from build123d import *

# Parameters (mm, degrees)
SKETCH1_W           = 36.310674736
SKETCH1_H           = 16.43794059
BOSS_EXTRUDE1_DEPTH = 2.54
FILLET1_R           = 2.54
FILLET2_R           = 2.54


# Some blends are built 0.0001 mm under size
with BuildPart() as part:
    # Sketch1 → Boss-Extrude1 (new body)
    with BuildSketch(Plane(origin=(0, 0, 0), x_dir=(1, 0, 0), z_dir=(0, 1, 0))):
        Rectangle(SKETCH1_W, SKETCH1_H)
    extrude(amount=BOSS_EXTRUDE1_DEPTH)

    # Fillet1
    fillet1_edges = [part.edges().sort_by_distance(p)[0] for p in [
        (18.155337368, 1.27, 8.218970295),
        (-18.155337368, 1.27, 8.218970295),
        (0, 2.54, 8.218970295),
    ]]
    fillet(fillet1_edges, radius=FILLET1_R - 0.0001)  # a hair under: the kernel refuses the full size

    # Fillet2
    # the kernel refuses this fillet: 2.54 mm, written as the material it takes off along each edge
    with BuildSketch(Plane(origin=(-15.615337368, 0, 8.218970295), x_dir=(0, 1, 0), z_dir=(1, 0, 0))) as fillet2_piece_1:
        with BuildLine():
            CenterArc((0.0001, -2.5399), 2.5399, 0, 90)
            Line((2.54, -2.5399), (2.54, 0))
            Line((2.54, 0), (0.0001, 0))
        make_face()
    revolve(axis=Axis((-15.615337368, 0, 8.218970295), (0, 0, 1)), revolution_arc=90, mode=Mode.SUBTRACT)
    with BuildSketch(Plane(origin=(15.615337368, 0, 8.218970295), x_dir=(1, 0, 0), z_dir=(0, -1, 0))) as fillet2_piece_2:
        with BuildLine():
            CenterArc((0.0001, -2.5399), 2.5399, 0, 90)
            Line((2.54, -2.5399), (2.54, 0))
            Line((2.54, 0), (0.0001, 0))
        make_face()
    revolve(axis=Axis((15.615337368, 0, 8.218970295), (0, 0, 1)), revolution_arc=90, mode=Mode.SUBTRACT)
    with BuildSketch(Plane(origin=(-18.155337368, 2.54, 8.218970295), x_dir=(0, -1, 0), z_dir=(0, 0, -1)), Plane(origin=(18.155337368, 2.54, -14.568970295), x_dir=(0, -1, 0), z_dir=(0, 0, 1))) as fillet2_piece_3:
        with BuildLine():
            CenterArc((FILLET2_R, -FILLET2_R), FILLET2_R, 90, 90)
            Line((0, -FILLET2_R), (0, 0))
            Line((0, 0), (FILLET2_R, 0))
        make_face()
    extrude(amount=22.78794059, mode=Mode.SUBTRACT)


solid = part.part
Could you check a few things on this model? Use its own coordinates, in mm. Give positions to 0.01 mm unless a question says otherwise; leave off trailing zeros. Write each loop counter-clockwise with the first axis right and the second up, starting at its lowest first coordinate (ties: lowest second). Pieces come first, ordered by that corner, then holes. Notation, with made-up numbers: (-1.75, 88.5) -> (14.25, 88.5) arc R18 cw to (14.25, 109.5) -> close; hole circle Ø7 at (18.5, 71). An arc over 180 degrees is marked (long way). Answer as CSV lines item,"result". Start each with the question number.
(1) Please list where these lines run through material, in increasing order: line 1 (Y direction, x = -15.5, z = 5.75); line 2 (Z direction, x = -9, y = 2.3); line 3 (Z direction, x = 1, y = 2.1).
(2) If we section it at B-B, the plane z = -6: Write out the boundary of the cut face in (x, y).
(3) I'm going to push flat-ended pins straight in: pin 1 Ø1.5 at (y, z) = (2.5, 2.5) entering from -X; pin 2 Ø1 at (x, y) = (3, 1.5) entering from +Z. Where does each tip first touch, or does it pass through?
Answer list:
1,line 1,"0 to 2.54"
1,line 2,"-8.22 to 6.76"
1,line 3,"-8.22 to 7.11"
2,outline,"(-18.16, 0) -> (18.16, 0) arc R2.54 ccw to (15.62, 2.54) -> (-15.62, 2.54) arc R2.54 ccw to start"
3,pin 1,"x = -17.46"
3,pin 2,"z = 8.01"
